For this review, take the finished solid that the model builds, in its own axes (mm). Face numbers are marked on the shaded views. Coordinates: 2 decimals unless noted, no trailing zeros. Loops run counter-clockwise (first coordinate to the right, second up) from the corner with the lowest first, then second, coordinate; pieces in that order, holes last. Notation, with made-up numbers: (-15.75, -26.5) - (15.25, -26.5) arc R29 cw to (15.25, -3.5) - close; hole circle Ø7 at (21.25, 56). An arc over 180 degrees is marked (long way). Use one line per item in the form item = value. Start each with the question number.
1. Draft analysis for pull direction Y (two halves, no side actions). For the marked faces 1, 2 and 3, state which applies: +Y half, -Y half, draft (parallel to the pull), parting line (faces both ways), or undercut.
2. Add section B-B on y = 0. Give the boundary of the cut face in (x, z) (3 decimals).
3. Add section D-D on x = 125. Give the boundary of the cut face in (y, z).
4. To check wall thickness, follow probe 1 along Y at (x, z) = (0, 9.25) (1 decimal); probe 2 along Y at (x, z) = (80, 13.3) (3 decimals); probe 3 along X at (y, z) = (0, 13.45) (3 decimals). State the ranges of each line that lie inside material, in increasing order.
5. For pin 1 Ø12 at (x, z) = (6, 4.5) entering from +Y; pin 2 Ø1 at (y, z) = (77, 6.5) entering from +X; pin 3 Ø6 at (x, z) = (14.5, 0.5) entering from -Y, all flat-tipped, find the tip position at first contact; note any pin that passes through.
6. Add section C-C on y = 156.5. Give the boundary of the cut face in (x, z), and give its area (3 significant figures).
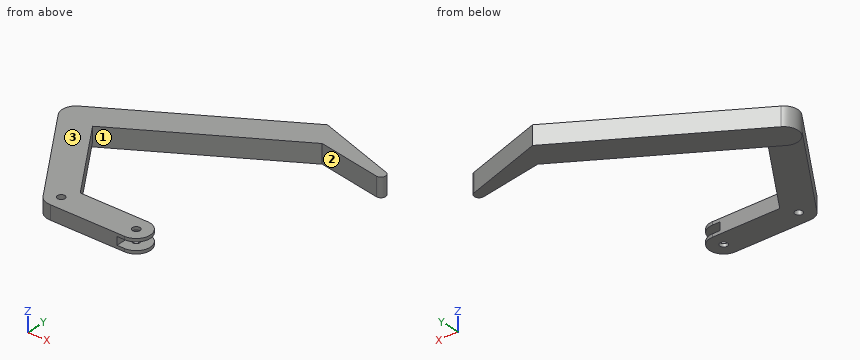
```python
from build123d import *

# Parameters (mm, degrees)
EXTRUDE_1_DEPTH          = 15
CUT_EXTRUDE_1_DEPTH      = 101.747208398
CUT_EXTRUDE_1_DEPTH_BACK = 101.747208398
SKETCH_2_W               = 23.23079143
SKETCH_2_H               = 8.5
CUT_EXTRUDE_2_DEPTH      = 98.33961167
CUT_EXTRUDE_2_DEPTH_BACK = 98.33961167
SKETCH_3_R               = 3.985
EXTRUDE_2_DEPTH          = 15
CUT_EXTRUDE_4_DEPTH      = 157.182605119
CUT_EXTRUDE_4_DEPTH_BACK = 157.182605119
SKETCH_9_R               = 3.985
CUT_EXTRUDE_5_DEPTH      = 157.182605119
CUT_EXTRUDE_5_DEPTH_BACK = 157.182605119
EXTRUDE_5_DEPTH          = 20
FILLET_1_R               = 5


with BuildPart() as part:
    # 草图1 → 凸台-拉伸1 (new body)
    with BuildSketch(Plane.XY):
        with BuildLine():
            Line((0, 15), (80, 15))
            ThreePointArc((80, 15), (95, 0), (80, -15))
            Line((80, -15), (0, -15))
            ThreePointArc((0, -15), (-15, 0), (0, 15))
        make_face()
    extrude(amount=EXTRUDE_1_DEPTH)

    # 草图2 → 切除-拉伸1 (cut, two sides: drawn at the far end of the back side and taken through both)
    with BuildSketch(Plane.XZ.offset(15).offset(-CUT_EXTRUDE_1_DEPTH_BACK)):
        with Locations((83.384604285, 7.5)):
            Rectangle(SKETCH_2_W, SKETCH_2_H)
    extrude(amount=CUT_EXTRUDE_1_DEPTH + CUT_EXTRUDE_1_DEPTH_BACK, mode=Mode.SUBTRACT)

    # 草图3 → 切除-拉伸2 (cut, two sides: drawn at the far end of the back side and taken through both)
    with BuildSketch(Plane(origin=(0, 0, 0), x_dir=(-1, 0, 0), z_dir=(0, 0, -1)).offset(-CUT_EXTRUDE_2_DEPTH_BACK)):
        with Locations((-80, 0)):
            Circle(SKETCH_3_R)
    extrude(amount=CUT_EXTRUDE_2_DEPTH + CUT_EXTRUDE_2_DEPTH_BACK, mode=Mode.SUBTRACT)

    # 草图4 → 凸台-拉伸2 (add)
    with BuildSketch(Plane.XY.offset(15)):
        with BuildLine():
            Line((-12.482779954, -8.354383615), (-84.788603834, 99.682035397))
            ThreePointArc((-84.788603834, 99.682035397), (-80.660207496, 120.519198965), (-59.823043927, 116.390802627))
            Line((-59.823043927, 116.390802627), (12.482779954, 8.354383615))
            ThreePointArc((12.482779954, 8.354383615), (8.354383615, -12.482779954), (-12.482779954, -8.354383615))
        make_face()
    extrude(amount=-EXTRUDE_2_DEPTH)

    # 草图9 → 切除-拉伸4 (cut, two sides: drawn at the far end of the back side and taken through both)
    with BuildSketch(Plane(origin=(0, 0, 0), x_dir=(-1, 0, 0), z_dir=(0, 0, -1)).offset(-CUT_EXTRUDE_4_DEPTH_BACK)):
        Circle(SKETCH_9_R)
    extrude(amount=CUT_EXTRUDE_4_DEPTH + CUT_EXTRUDE_4_DEPTH_BACK, mode=Mode.SUBTRACT)

    # 草图10 → 切除-拉伸5 (cut, two sides: drawn at the far end of the back side and taken through both)
    with BuildSketch(Plane.XY.offset(15).offset(-CUT_EXTRUDE_5_DEPTH_BACK)):
        Polygon((-84.788603834, 99.682035397), (-48.234850364, 123.999680139), (-59.64356033, 141.14900426), (-100.506345589, 113.964745441), (-89.097635623, 96.815421321), align=None)
    extrude(amount=CUT_EXTRUDE_5_DEPTH + CUT_EXTRUDE_5_DEPTH_BACK, mode=Mode.SUBTRACT)

    # 草图11 → 凸台-拉伸5 (add)
    with BuildSketch(Plane.XY.offset(15)):
        with BuildLine():
            Line((97.484212933, 227.748715927), (249.011128895, 178.572894151))
            Line((249.011128895, 178.572894151), (112.956276539, 202.05846487))
            Line((112.956276539, 202.05846487), (-64.546579612, 95.156610362))
            ThreePointArc((-64.546579612, 95.156610362), (-85.127736943, 100.265704087), (-80.018643218, 120.846861419))
            Line((-80.018643218, 120.846861419), (97.484212933, 227.748715927))
        make_face()
    extrude(amount=-EXTRUDE_5_DEPTH)

    # 圆角1
    fillet_1_edges = [part.edges().sort_by_distance(p)[0] for p in [
        (249.011128895, 178.572894151, 5),
    ]]
    fillet(fillet_1_edges, radius=FILLET_1_R)


solid = part.part
```
Conclusion:
q1.face_1 = undercut
q1.face_2 = -Y half
q1.face_3 = draft
q2.outline = (-18.074, 0) - (-3.985, 0) - (-3.985, 15) - (-18.074, 15) - close; (3.985, 0) - (76.015, 0) - (76.015, 3.25) - (71.769, 3.25) - (71.769, 11.75) - (76.015, 11.75) - (76.015, 15) - (3.985, 15) - close; (83.985, 0) - (95, 0) - (95, 3.25) - (83.985, 3.25) - close; (83.985, 11.75) - (95, 11.75) - (95, 15) - (83.985, 15) - close
q3.outline = (199.98, -5) - (218.82, -5) - (218.82, 15) - (199.98, 15) - close
q4.probe_1 = -15 to -4, 4 to 27, 134 to 169
q4.probe_2 = -15 to -3.985, 3.985 to 15, 182.21 to 217.219
q4.probe_3 = -18.074 to -3.985, 3.985 to 76.015, 83.985 to 95
q5.pin_1 = 176.27
q5.pin_2 = -33.13
q5.pin_3 = -15
q6.outline = (-20.82, -5) - (37.31, -5) - (37.31, 15) - (-20.82, 15) - close
q6.area = 1,160 mm^2
